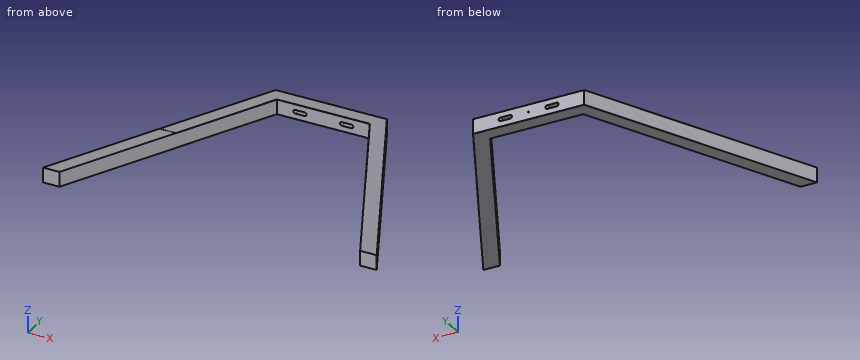
Autodesk Inventor part; units mm, degrees
ref_plane "YZ Plane" through (0, 0, 0) normal (1, 0, 0) x (0, 1, 0)
ref_plane "XZ Plane" through (0, 0, 0) normal (0, 1, 0) x (-1, 0, 0)
ref_plane "XY Plane" through (0, 0, 0) normal (0, 0, 1) x (1, 0, 0)
sketch "Sketch1" plane through (0, 0, 0) normal (0, 0, 1) x (1, 0, 0)
  line L0 (9.7407, 1114.2593) -> (159.7407, 1114.2593)
  line L1 (9.7407, 1114.2593) -> (-140.2593, 1114.2593)
  line L2 (-290.2593, 814.2593) -> (-140.2593, 1114.2593)
  line L3 (159.7407, 1114.2593) -> (459.7407, 514.2593)
  line L4 (135.0194, 1074.2593) -> (9.7407, 1074.2593)
  line L5 (9.7407, 1074.2593) -> (-115.5379, 1074.2593)
  line L6 (-115.5379, 1074.2593) -> (-245.5379, 814.2593)
  line L7 (9.7407, 1114.2593) -> (159.7407, 1114.2593)
  line L8 (9.7407, 1114.2593) -> (-140.2593, 1114.2593)
  line L9 (-440.2593, 514.2593) -> (-140.2593, 1114.2593)
  line L10 (159.7407, 1114.2593) -> (309.9483, 813.8441)
  line L11 (135.0194, 1074.2593) -> (9.7407, 1074.2593)
  line L12 (9.7407, 1074.2593) -> (-115.5379, 1074.2593)
  line L13 (-115.5379, 1074.2593) -> (-245.5379, 814.2593)
  line L14 (-245.5379, 814.2593) -> (-290.2593, 814.2593)
  line L15 (265.227, 813.8441) -> (309.9483, 813.8441)
  line L16 (265.227, 813.8441) -> (135.0194, 1074.2593)
  line L17 (415.0194, 514.2593) -> (135.0194, 1074.2593)
  line L18 (-395.5379, 514.2593) -> (-440.2593, 514.2593)
  line L19 (-245.5379, 814.2593) -> (-395.5379, 514.2593)
  line L20 (-440.2593, 514.2593) -> (-395.5379, 514.2593)
  line L21 (415.0194, 514.2593) -> (459.7407, 514.2593)
  point P0 (0, 0)
  dimension "d13" = 300
extrude "Extrusion1" add sketch "Sketch1" along normal blind 40 contours L0 L3 L15 L16 L4 L5 L6 L14 L2 L1
fillet "Fillet1" radius 0.5 10 edges at (72.3801, 1074.2593, 40) (72.3801, 1074.2593, 0) (200.1232, 944.0517, 40) (234.8445, 964.0517, 40) (-65.2593, 1114.2593, 40) (-215.2593, 964.2593, 40) (-180.5379, 944.2593, 40) (-267.8986, 814.2593, 40) (-180.5379, 944.2593, 0) (234.8445, 964.0517, 0)
fillet "Fillet2" radius 0.5 1 edges at (200.1232, 944.0517, 0)
fillet "Fillet3" radius 0.5 3 edges at (159.7407, 1114.2593, 20) (84.4612, 1114.2593, 0) (-215.2593, 964.2593, 0)
sketch "Sketch2" plane through (-140.2593, 1114.2593, 0.5) normal (0, 1, 0) x (1, 0, 0)
  line L0 (300.1382, -39) -> (300.1382, 0)
  line L1 (300.1382, -19.5) -> (0, -19.5)
  line L2 (0, 0) -> (0, -39)
  circle A0 centre (150.0691, -19.5) radius 1.5
  point P0 (140.2593, 0.5)
  dimension "d14" = 3
extrude "Extrusion2" cut sketch "Sketch2" against normal blind 10
extrude "Extrusion3" add sketch "Sketch1" along normal blind 40 contours L3 L21 L17 L15 | L14 L19 L18 L9
sketch "Sketch3" plane through (-140.2593, 1114.2593, 0.5) normal (0, 1, 0) x (1, 0, 0)
  point P0 (140.2593, 0.5)
sketch "Sketch4" plane through (-140.2593, 1114.2593, 0.5) normal (0, 1, 0) x (1, 0, 0)
  circle A0 centre (150.0691, -19.5) radius 1.5
  line L0 (0, 0) -> (299.691, 0)
  line L1 (0, 0) -> (0, -39)
  line L2 (299.691, -39) -> (0, -39)
  line L3 (299.691, 0) -> (299.691, -39)
  line L4 (200.1691, -14.5) -> (225.9691, -14.5)
  line L5 (225.9691, -24.5) -> (200.1691, -24.5)
  arc A1 (225.9691, -24.5) -> (225.9691, -14.5) centre (225.9691, -19.5) ccw
  arc A2 (200.1691, -14.5) -> (200.1691, -24.5) centre (200.1691, -19.5) ccw
  arc A3 (74.1691, -14.5) -> (74.1691, -24.5) centre (74.1691, -19.5) ccw
  line L6 (74.1691, -14.5) -> (99.9691, -14.5)
  line L7 (74.1691, -24.5) -> (99.9691, -24.5)
  arc A4 (99.9691, -24.5) -> (99.9691, -14.5) centre (99.9691, -19.5) ccw
  point P0 (140.2593, 0.5)
extrude "Extrusion4" cut sketch "Sketch4" against normal blind 50 contours L4 A1 L5 A2 | L6 A4 L7 A3
properties part number "CAVALETE_INFERIOR" material "SAE 1010/1020"
Part model, mm, in its own coordinate system. Coordinates: 2 decimals unless noted, no trailing zeros. Write each loop counter-clockwise with the first axis right and the second up, starting at its lowest first coordinate (ties: lowest second). Pieces come first, ordered by that corner, then holes. Notation, with made-up numbers: (-23, -38.75) - (-8, -38.75) arc R6 cw to (-8, -33.75) - close; hole circle Ø7 at (-9, 4.5). An arc over 180 degrees is marked (long way). Put each result on its own line as item: value.
1. Band-saw the part on A-A (y = 620). Write the cut outline in (x, z), then the cut area to 3 significant figures.
Final values:
outline: (-387.39, 0) - (-342.67, 0) - (-342.67, 40) - (-387.39, 40) - close; (362.15, 0) - (406.87, 0) - (406.87, 40) - (362.15, 40) - close
area: 3,580 mm²
2. Band-saw the part on B-B (x = 351.5). Write the cut outline in (y, z).
Final values:
outline: (641.3, 0) - (730.74, 0) - (730.74, 40) - (641.3, 40) - close
3. Probe line 1 along X through (y, z) = (1106, 20); line 2 along X through (y, z) = (1106.75, 20); line 3 along X through (y, z) = (587.5, 8). List the from-to ranges inside material, lowest first. Write a range as [from, to].
Final values:
line 1: x = [-144.39, -71.09], [-35.29, 8.31], [11.31, 54.91], [90.71, 163.87]
line 2: x = [-144.01, -71.09], [-35.29, 8.31], [11.31, 54.91], [90.71, 163.5]
line 3: x = [-403.64, -358.92], [378.4, 423.12]
4. Flat gauge pins, fed straight in: pin 1 Ø8 at (x, z) = (-312.5, 34.5) entering from +Y; pin 2 Ø1.5 at (x, z) = (22.5, 34.5) entering from -Y; pin 3 Ø8 at (x, z) = (325, 11.5) entering from -Y. Where does each tip first touch, or does it go through?
Final values:
pin 1: stops at y = 777.78
pin 2: stops at y = 1074.26
pin 3: stops at y = 686.3
